```python
from build123d import *

# Parameters (mm, degrees)
SKETCH1_R           = 125
SKETCH1_R_2         = 50
BOSS_EXTRUDE1_DEPTH = 50
SKETCH2_W           = 40
SKETCH2_H           = 30
CUT_EXTRUDE1_DEPTH  = 1
CIRPATTERN1_COUNT   = 8


with BuildPart() as part:
    # Sketch1 → Boss-Extrude1 (new, symmetric)
    with BuildSketch(Plane(origin=(0, 0, 0), x_dir=(1, 0, 0), z_dir=(0, 1, 0))):
        with Locations(Location((0, 0, 0), (0, 0, 270))):
            Circle(SKETCH1_R)
        with Locations(Location((0, 0, 0), (0, 0, 270))):
            Circle(SKETCH1_R_2, mode=Mode.SUBTRACT)
    extrude(amount=BOSS_EXTRUDE1_DEPTH, both=True)

    # Sketch2 → Cut-Extrude1 (cut)
    with BuildSketch(Plane(origin=(0, 50, 0), x_dir=(1, 0, 0), z_dir=(0, 1, 0))):
        with Locations((0, 85)):
            Rectangle(SKETCH2_W, SKETCH2_H)
    cut_extrude1 = extrude(amount=-CUT_EXTRUDE1_DEPTH, mode=Mode.SUBTRACT)

    # CirPattern1: Cut-Extrude1 ×8 about axis
    cirpattern1_axis = Axis((0, 0, 0), (0, 1, 0))
    for i in range(1, CIRPATTERN1_COUNT):
        add(cut_extrude1.rotate(cirpattern1_axis, i * 360 / CIRPATTERN1_COUNT), mode=Mode.SUBTRACT)


solid = part.part
```
Model file for the job. Use its own axes, mm. A direction names the side the tool comes from. Coordinates: 2 decimals unless noted, no trailing zeros. Write each loop counter-clockwise with the first axis right and the second up, starting at its lowest first coordinate (ties: lowest second). Pieces come first, ordered by that corner, then holes. Notation, with made-up numbers: (39.25, -35.75) - (81.25, -35.75) arc R18 ccw to (81.25, -29.75) - close; hole circle Ø3 at (-28.5, -19.75). An arc over 180 degrees is marked (long way). Use a Markdown table: item, result. Add a question column.
Item 1: Band-saw the part on B-B, the plane x = 0. Write the cut outline in (y, z).
Item 2: 3-axis set-ups, long thin cutter, end or side, ignore diameter. For faces 5 (the face through (2, 50, 54)), 6 (the face through (45.813, 49.507, -74.098)): which of +Z, -Z, +X, -X, +Y, -Y reach the whole face in a straight line?
Item 3: Drill centre lines: line 1 along X through (y, z) = (10, 0); line 2 along Y through (x, z) = (-52, 52); line 3 along Z through (x, y) = (-2.5, -30) (3 decimals). Where is each one in solid material? Low to high.
Item 4: Two-plate mould, pull along Z, no slides. Class faces 1 (the face through (-54, -50, -2)), 2 (the face through (70.91, 49.51, 70.51)), 3 (the face through (70.51, 49.51, -70.91)), 4 (the face through (5.5, 0.7, -124.88)): pulls with the +Z half, pulls with the -Z half, needs draft (parallel to the pull), parting line crosses it, or undercut.
Item 5: Drop flat-ended pins along their axis: pin 1 (10 mm diameter, centred on x = 47.5, y = 22, fed in from +Z); pin 2 (10 mm diameter, centred on y = 0.5, z = -55, fed in from -X); pin 3 (0.8 mm diameter, centred on y = 49.5, z = 86, fed in from -X). Give the stop position or say it passes through.
Item 6: Band-saw the part on D-D, the plane y = 39.5. Write the cut outline in (x, z), and give its area (3 significant figures).
Item 7: Band-saw the part on A-A, the plane z = 0. Write the cut outline in (x, y), and give its area (3 significant figures).
Item 8: Band-saw the part on C-C, the plane x = 74.5. Write the cut outline in (y, z), and give its area (3 significant figures).
A:
| question | item | result |
|---|---|---|
| 1 | outline | (-50, -125) - (50, -125) - (50, -100) - (49, -100) - (49, -70) - (50, -70) - (50, -50) - (-50, -50) - close; (-50, 50) - (50, 50) - (50, 70) - (49, 70) - (49, 100) - (50, 100) - (50, 125) - (-50, 125) - close |
| 2 | face 5 | +Z, -Z, +X, -X, +Y |
| 2 | face 6 | +Y |
| 3 | line 1 | x = -125 to -50, 50 to 125 |
| 3 | line 2 | y = -50 to 49 |
| 3 | line 3 | z = -124.975 to -49.937, 49.937 to 124.975 |
| 4 | face 1 | needs draft |
| 4 | face 2 | undercut |
| 4 | face 3 | undercut |
| 4 | face 4 | parting line crosses it |
| 5 | pin 1 | stops at z = 117.55 |
| 5 | pin 2 | stops at x = -114.56 |
| 5 | pin 3 | stops at x = -91.09 |
| 6 | outline | circle Ø250 at (0, 0); hole circle Ø100 at (0, 0) |
| 6 | area | 41,200 mm² |
| 7 | outline | (-125, -50) - (-50, -50) - (-50, 50) - (-70, 50) - (-70, 49) - (-100, 49) - (-100, 50) - (-125, 50) - close; (50, -50) - (125, -50) - (125, 50) - (100, 50) - (100, 49) - (70, 49) - (70, 50) - (50, 50) - close |
| 7 | area | 14,900 mm² |
| 8 | outline | (-50, -100.37) - (50, -100.37) - (50, -66.92) - (49, -66.92) - (49, -46.22) - (50, -46.22) - (50, -20) - (49, -20) - (49, 20) - (50, 20) - (50, 46.22) - (49, 46.22) - (49, 66.92) - (50, 66.92) - (50, 100.37) - (-50, 100.37) - close |
| 8 | area | 20,000 mm² |
